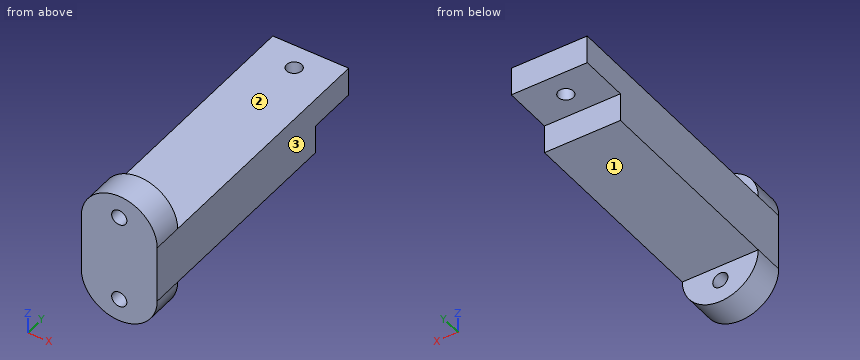
```python
from build123d import *

# Parameters (mm, degrees)
SKETCH1_W           = 20
SKETCH1_H           = 75
BOSS_EXTRUDE1_DEPTH = 15
SKETCH2_R           = 2
BOSS_EXTRUDE2_DEPTH = 8
SKETCH3_W           = 20
SKETCH3_H           = 7.5
CUT_EXTRUDE1_DEPTH  = 13
SKETCH4_R           = 2
CUT_EXTRUDE2_DEPTH  = 13


with BuildPart() as part:
    # Sketch1 → Boss-Extrude1 (new body)
    with BuildSketch(Plane.XY):
        Rectangle(SKETCH1_W, SKETCH1_H)
    extrude(amount=BOSS_EXTRUDE1_DEPTH)

    # Sketch2 → Boss-Extrude2 (add)
    # profile 1 of 2: a face of its own
    with BuildSketch(Plane.XZ.offset(37.5)):
        with BuildLine():
            Line((-10, 0), (10, 0))
            ThreePointArc((10, 0), (0, -10), (-10, 0))
        make_face()
        with Locations(Location((0, -4, 0), (0, 0, 270))):
            Circle(SKETCH2_R, mode=Mode.SUBTRACT)
    # profile 2 of 2: a face of its own
    with BuildSketch(Plane.XZ.offset(37.5)):
        with BuildLine():
            Line((-10, 15), (10, 15))
            ThreePointArc((10, 15), (0, 25), (-10, 15))
        make_face()
        with Locations(Location((0, 19, 0), (0, 0, 90))):
            Circle(SKETCH2_R, mode=Mode.SUBTRACT)
    extrude(amount=-BOSS_EXTRUDE2_DEPTH)

    # Sketch3 → Cut-Extrude1 (cut)
    with BuildSketch(Plane(origin=(0, 37.5, 0), x_dir=(1, 0, 0), z_dir=(0, 1, 0))):
        with Locations((0, -3.75)):
            Rectangle(SKETCH3_W, SKETCH3_H)
    extrude(amount=-CUT_EXTRUDE1_DEPTH, mode=Mode.SUBTRACT)

    # Sketch4 → Cut-Extrude2 (cut)
    with BuildSketch(Plane(origin=(0, 0, 7.5), x_dir=(-1, 0, 0), z_dir=(0, 0, -1))):
        with Locations((0, 31)):
            Circle(SKETCH4_R)
    extrude(amount=-CUT_EXTRUDE2_DEPTH, mode=Mode.SUBTRACT)


solid = part.part
```
Can you work these out from the model? Positions are in its coordinate system, mm. Face numbers are marked on the shaded views. A direction names the side the tool comes from. Coordinates: 2 decimals unless noted, no trailing zeros. Write each loop counter-clockwise with the first axis right and the second up, starting at its lowest first coordinate (ties: lowest second). Pieces come first, ordered by that corner, then holes. Notation, with made-up numbers: (69, -26.5) - (103, -26.5) arc R24 ccw to (103, -3.5) - close; hole circle Ø5 at (7.5, 17.5). An arc over 180 degrees is marked (long way). Return JSON: item names as keys, results as strings.
Q1. If we section it at D-D (x = 8.5): Please give me the cut outline in (y, z), then the cut area to 3 significant figures.
Computed values:
{"outline": "(-37.5, -5.27) - (-29.5, -5.27) - (-29.5, 0) - (24.5, 0) - (24.5, 7.5) - (37.5, 7.5) - (37.5, 15) - (-29.5, 15) - (-29.5, 20.27) - (-37.5, 20.27) - close", "area": "1,110 mm2"}
Q2. On a 3-axis mill with a long thin cutter (end or side, diameter ignored), from which of +Z, -Z, +X, -X, +Y, -Y can I reach the whole of each face in a straight line? I mean the marked faces 1, 2 and 3. Say none if no direction works.
Computed values:
{"face 1": "-Z, +X, -X, +Y", "face 2": "+Z, +X, -X, +Y", "face 3": "+Z, -Z, +X, +Y, -Y"}
Q3. If we section it at B-B (y = 31): Please give me the cut outline in (x, z), then the cut area to 3 significant figures.
Computed values:
{"outline": "(-10, 7.5) - (-2, 7.5) - (-2, 15) - (-10, 15) - close; (2, 7.5) - (10, 7.5) - (10, 15) - (2, 15) - close", "area": "120 mm2"}
Q4. If we section it at A-A (x = 0): Please give me the cut outline in (y, z).
Computed values:
{"outline": "(-37.5, -10) - (-29.5, -10) - (-29.5, -6) - (-37.5, -6) - close; (-37.5, -2) - (-29.5, -2) - (-29.5, 0) - (24.5, 0) - (24.5, 7.5) - (29, 7.5) - (29, 15) - (-29.5, 15) - (-29.5, 17) - (-37.5, 17) - close; (-37.5, 21) - (-29.5, 21) - (-29.5, 25) - (-37.5, 25) - close; (33, 7.5) - (37.5, 7.5) - (37.5, 15) - (33, 15) - close"}
Q5. I'm going to push flat-ended pins straight in: pin 1 Ø4 at (y, z) = (26.5, -0.5) entering from +X; pin 2 Ø4 at (x, y) = (2.5, -22.5) entering from +Z; pin 3 Ø8 at (x, z) = (-2.5, 20.5) entering from +Y; pin 4 Ø4 at (x, y) = (1, 28.5) entering from -Z. Where does each tip first touch, or does it pass through?
Computed values:
{"pin 1": "passes through", "pin 2": "stops at z = 15", "pin 3": "stops at y = -29.5", "pin 4": "stops at z = 7.5"}
Q6. Please list where these lines run through material, in increasing order: L1, parallel to Y at x = 0.25, z = 11; L2, parallel to Z at x = 7.75, y = 33; L3, parallel to Y at x = -4.5, z = -1. Write a range as from..to.
Computed values:
{"L1": "y = -37.5..29.02, 32.98..37.5", "L2": "z = 7.5..15", "L3": "y = -37.5..-29.5"}
Q7. If we section it at C-C (z = 19): Please give me the cut outline in (x, y), then the cut area to 3 significant figures.
Computed values:
{"outline": "(-9.17, -37.5) - (-2, -37.5) - (-2, -29.5) - (-9.17, -29.5) - close; (2, -37.5) - (9.17, -37.5) - (9.17, -29.5) - (2, -29.5) - close", "area": "115 mm2"}
